```python
from build123d import *

# Parameters (mm, degrees)
SKETCH2_W           = 4.7625
SKETCH2_H           = 44.223214285
SKETCH2_H_2         = 44.223214286
SKETCH2_W_2         = 21.998214286
SKETCH2_H_3         = 4.7625
SKETCH2_W_3         = 26.760714286
BOSS_EXTRUDE1_DEPTH = 4.7625
SKETCH3_W           = 7.9375
SKETCH3_H           = 228.6
CUT_EXTRUDE1_DEPTH  = 184.017476539
SKETCH4_R           = 3.175
CUT_EXTRUDE2_DEPTH  = 184.017476539


with BuildPart() as part:
    # Sketch2 → Boss-Extrude1 (new body)
    with BuildSketch(Plane.XY):
        Polygon((0, -152.4), (0, 152.4), (-88.9, 152.4), (-88.9, 108.176785714), (-88.9, 63.953571429), (-88.9, 19.730357143), (-88.9, -24.492857143), (-88.9, -68.716071429), (-88.9, -112.939285714), (-88.9, -152.4), (-66.901785714, -152.4), (-40.141071429, -152.4), (-13.380357143, -152.4), align=None)
        Polygon((88.9, 152.4), (0, 152.4), (0, -152.4), (13.380357143, -152.4), (40.141071429, -152.4), (66.901785714, -152.4), (88.9, -152.4), (88.9, -112.939285714), (88.9, -68.716071429), (88.9, -24.492857143), (88.9, 19.730357143), (88.9, 63.953571429), (88.9, 108.176785714), align=None)
        with Locations((-91.28125, 86.065178572)):
            Rectangle(SKETCH2_W, SKETCH2_H)
        with Locations((-91.28125, -2.38125)):
            Rectangle(SKETCH2_W, SKETCH2_H_2)
        with Locations((-91.28125, -90.827678572)):
            Rectangle(SKETCH2_W, SKETCH2_H)
        with Locations((-77.900892857, -154.78125)):
            Rectangle(SKETCH2_W_2, SKETCH2_H_3)
        with Locations((-26.760714286, -154.78125)):
            Rectangle(SKETCH2_W_3, SKETCH2_H_3)
        with Locations((26.760714286, -154.78125)):
            Rectangle(SKETCH2_W_3, SKETCH2_H_3)
        with Locations((91.28125, -90.827678572)):
            Rectangle(SKETCH2_W, SKETCH2_H)
        with Locations((91.28125, -2.38125)):
            Rectangle(SKETCH2_W, SKETCH2_H_2)
        with Locations((91.28125, 86.065178572)):
            Rectangle(SKETCH2_W, SKETCH2_H)
        with Locations((77.900892857, -154.78125)):
            Rectangle(SKETCH2_W_2, SKETCH2_H_3)
    extrude(amount=BOSS_EXTRUDE1_DEPTH)

    # Sketch3 → Cut-Extrude1 (cut, through all)
    with BuildSketch(Plane.XY.offset(4.7625)):
        with Locations((0, 38.1)):
            Rectangle(SKETCH3_W, SKETCH3_H)
    extrude(amount=-CUT_EXTRUDE1_DEPTH, mode=Mode.SUBTRACT)

    # Sketch4 → Cut-Extrude2 (cut, through all)
    with BuildSketch(Plane.XY.offset(4.7625)):
        with Locations((-50.8, -139.7)):
            Circle(SKETCH4_R)
    extrude(amount=-CUT_EXTRUDE2_DEPTH, mode=Mode.SUBTRACT)


solid = part.part
```
Input: part model. Units: mm. Frame: model coordinates. Coordinates: 2 decimals unless noted, no trailing zeros. Loops run counter-clockwise (first coordinate to the right, second up) from the corner with the lowest first, then second, coordinate; pieces in that order, holes last. Notation, with made-up numbers: (41, 64.25) -> (74, 64.25) arc R20 cw to (74, 101.25) -> close; hole circle Ø4 at (21, 69.25). An arc over 180 degrees is marked (long way). Use a Markdown table: item, result.
1) Contact query for flat-ended pins moving along their axis: pin 1 (1 mm diameter, centred on y = 44.5, z = 1.5, fed in from -X); pin 2 (2.5 mm diameter, centred on x = -92, z = 3.5, fed in from -Y); pin 3 (2.5 mm diameter, centred on y = -155.5, z = 2.5, fed in from +X). Output: stop coordinate, or through.
Results found:
| item | result |
|---|---|
| pin 1 | stops at x = -88.9 |
| pin 2 | stops at y = -112.94 |
| pin 3 | stops at x = 88.9 |
2) Cut plane A-A (x = -50.8). Return the cut outline in (y, z) (1 decimal), then the cut area to 3 significant figures.
Results found:
| item | result |
|---|---|
| outline | (-152.4, 0) -> (-142.9, 0) -> (-142.9, 4.8) -> (-152.4, 4.8) -> close; (-136.5, 0) -> (152.4, 0) -> (152.4, 4.8) -> (-136.5, 4.8) -> close |
| area | 1,420 mm2 |
3) Pull-direction query (X, two-part tool) for faces 1 (the cylindrical face through (-51.21, -136.55, 2.41)), 2 (the flat face through (-22, 0, 4.762)); classes: released by +X, released by -X, zero draft, split by the parting line, or undercut.
Results found:
| item | result |
|---|---|
| face 1 | undercut |
| face 2 | zero draft |
4) Cut plane B-B (y = -139.7). Return the cut outline in (x, z) (1 decimal).
Results found:
| item | result |
|---|---|
| outline | (-88.9, 0) -> (-54, 0) -> (-54, 4.8) -> (-88.9, 4.8) -> close; (-47.6, 0) -> (88.9, 0) -> (88.9, 4.8) -> (-47.6, 4.8) -> close |
5) Material intervals for line 1 along Y through (x, z) = (-50.8, 3.15) (3 decimals); line 2 along X through (y, z) = (-139.7, 1.6) (3 decimals); line 3 along X through (y, z) = (128, 0.5), sorted ascending. Write a range as from..to.
Results found:
| item | result |
|---|---|
| line 1 | y = -152.4..-142.875, -136.525..152.4 |
| line 2 | x = -88.9..-53.975, -47.625..88.9 |
| line 3 | x = -88.9..-3.97, 3.97..88.9 |
